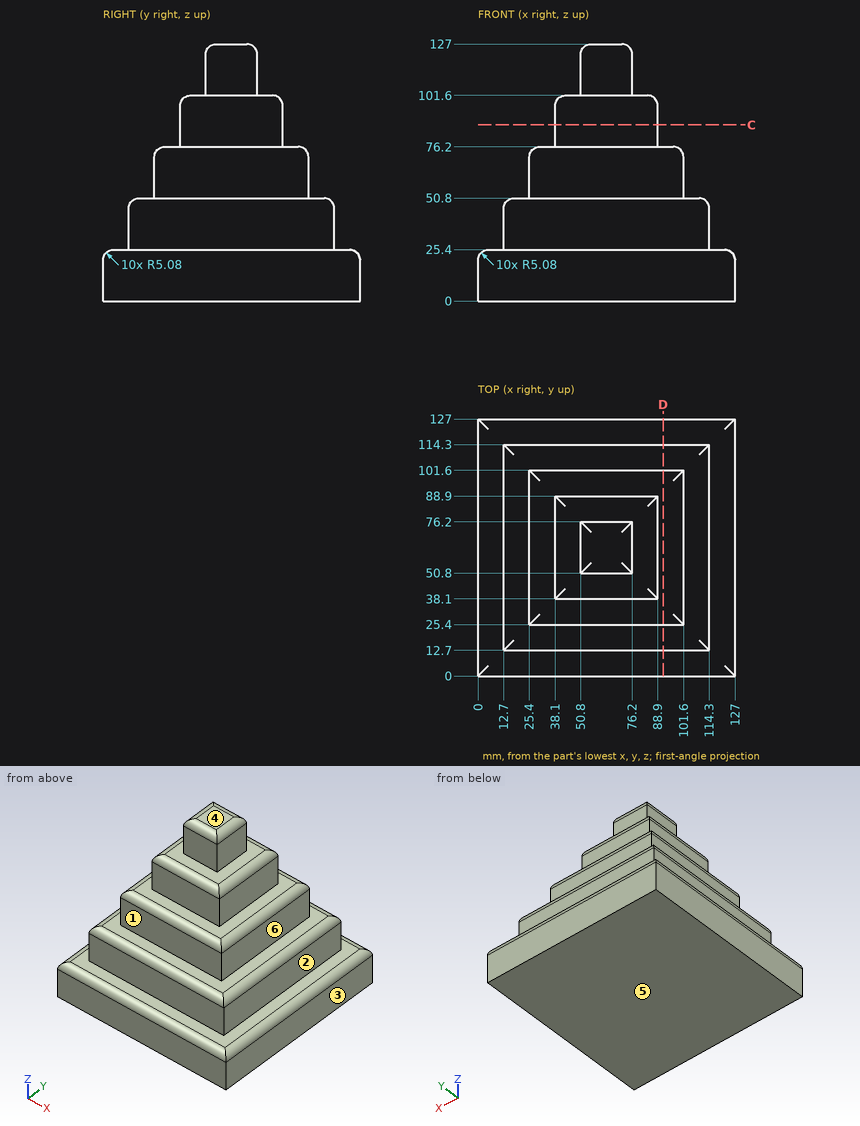
The figure shows three views and two pictorial views of one solid part (mm, origin at its lowest corner). Answer the questions. A direction names the side the tool comes from. Give positions to 0.01 mm unless a question says otherwise; leave off trailing zeros. Order: outer loops, then holes, each group sorted by start corner. A loop starts at its lowest first (then second) coordinate and runs counter-clockwise, first axis right, second up. Notation, with made-up numbers: (18, 77.5) - (66, 77.5) arc R28 cw to (66, 102.5) - close; hole circle Ø7 at (86, 34). An arc over 180 degrees is marked (long way). Answer as CSV lines item,"result".
Q1. Determine the mould class of the marked faces 4, 5 and 6 for opening direction Z: pulls with the +Z half, pulls with the -Z half, needs draft (parallel to the pull), parting line crosses it, or undercut.
Answer key:
face 4,"pulls with the +Z half"
face 5,"pulls with the -Z half"
face 6,"needs draft"
Q2. Which of the six approach directions +Z, -Z, +X, -X, +Y, -Y give full straight-line access (tool end or side, diameter ignored) to the marked faces 1, 2 and 3?
Answer key:
face 1,"+Z, +X, -X, -Y"
face 2,"+Z, +X, +Y, -Y"
face 3,"+Z, -Z, +X, +Y, -Y"
Q3. Each of these flat-tipped pins is pushed along its axis until it touches: pin 1 Ø8 at (x, y) = (98, 91) entering from -Z; pin 2 Ø22.5 at (x, z) = (66, 113.5) entering from -Y; pin 3 Ø16.5 at (y, z) = (62, 82.5) entering from +X; pin 4 Ø2 at (x, y) = (32, 26) entering from +Z. Where does it stop, or does it pass through?
Answer key:
pin 1,"stops at z = 0"
pin 2,"stops at y = 50.8"
pin 3,"stops at x = 100.52"
pin 4,"stops at z = 74.82"
Q4. A cutting plane is placed at D-D, the plane x = 91.5. Determine the outline of the cut face in (y, z), and give its area (3 significant figures).
Answer key:
outline,"(0, 0) - (127, 0) - (127, 20.32) arc R5.08 ccw to (121.92, 25.4) - (114.3, 25.4) - (114.3, 45.72) arc R5.08 ccw to (109.22, 50.8) - (101.6, 50.8) - (101.6, 71.12) arc R5.08 ccw to (96.52, 76.2) - (30.48, 76.2) arc R5.08 ccw to (25.4, 71.12) - (25.4, 50.8) - (17.78, 50.8) arc R5.08 ccw to (12.7, 45.72) - (12.7, 25.4) - (5.08, 25.4) arc R5.08 ccw to (0, 20.32) - close"
area,"7,710 mm^2"
Q5. Straight lines are drawn through the part: L1, parallel to Z at x = 121, y = 25; L2, parallel to X at y = 21, z = 41; L3, parallel to Y at x = 47, z = 89. For each, find the intervals that lie inside material, in ascending order.
Answer key:
L1,"z = 0 to 25.4"
L2,"x = 12.7 to 114.3"
L3,"y = 38.1 to 88.9"
Q6. A cutting plane is placed at C-C, the plane z = 87. Determine the outline of the cut face in (x, y), and give its area (3 significant figures).
Answer key:
outline,"(38.1, 38.1) - (88.9, 38.1) - (88.9, 88.9) - (38.1, 88.9) - close"
area,"2,580 mm^2"
